Input: dimensioned drawing with shaded views. Units: mm. Origin: part minimum x, y, z. Give positions to 0.01 mm unless a question says otherwise; leave off trailing zeros. Write each loop counter-clockwise with the first axis right and the second up, starting at its lowest first coordinate (ties: lowest second). Pieces come first, ordered by that corner, then holes. Notation, with made-up numbers: (-7, 54.5) -> (10, 54.5) arc R22 ccw to (10, 84.5) -> close; hole circle Ø1 at (62.25, 53.5). An arc over 180 degrees is marked (long way). Answer as a JSON object with one key per item and string values.
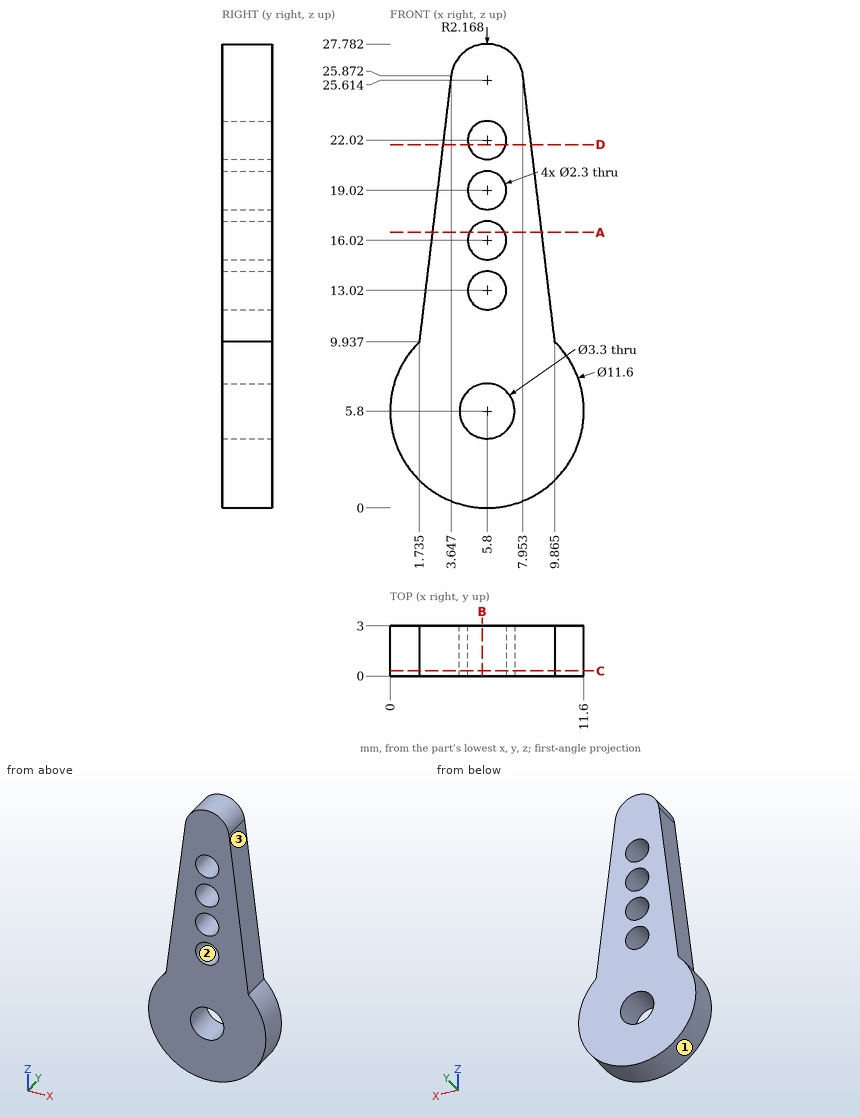
Q1. First-contact query: P1, Ø1.8, axis at x = 5.8, z = 16.02, coming from the -Y side; P2, Ø3.5, axis at x = 5.8, z = 13.02, coming from the -Y side. Flat tips, straight axial feed; report the tip coordinate or a pass-through.
Values:
{"P1": "through", "P2": "y = 0"}
Q2. Material intervals for L1, parallel to Z at x = 5.75, y = 2.35; L2, parallel to Z at x = 7, y = 1.8 (1 decimal); L3, parallel to X at y = 1.8, z = 21.75, sorted ascending. Write a range as from..to.
Values:
{"L1": "0..4.15, 7.45..11.87, 14.17..14.87, 17.17..17.87, 20.17..20.87, 23.17..27.78", "L2": "0.1..4.7, 6.9..27.4", "L3": "3.15..4.68, 6.92..8.45"}
Q3. Mould query, pull axis X, two halves, no side actions, for the marked faces 1, 2 and 3. Classes: pulls with the +X half, pulls with the -X half, needs draft (parallel to the pull), parting line crosses it, or undercut.
Values:
{"face 1": "parting line crosses it", "face 2": "undercut", "face 3": "pulls with the +X half"}
Q4. Cut plane D-D (z = 21.75). Return the cut outline in (x, y).
Values:
{"outline": "(3.15, 0) -> (4.68, 0) -> (4.68, 3) -> (3.15, 3) -> close; (6.92, 0) -> (8.45, 0) -> (8.45, 3) -> (6.92, 3) -> close"}
Q5. Cut plane A-A (z = 16.5). Return the cut outline in (x, y) (1 decimal), and give its area (3 significant figures).
Values:
{"outline": "(2.5, 0) -> (4.8, 0) -> (4.8, 3) -> (2.5, 3) -> close; (6.8, 0) -> (9.1, 0) -> (9.1, 3) -> (6.8, 3) -> close", "area": "13.4 mm²"}
Q6. Cut plane B-B (x = 5.5). Return the cut outline in (y, z).
Values:
{"outline": "(0, 0.01) -> (3, 0.01) -> (3, 4.18) -> (0, 4.18) -> close; (0, 7.42) -> (3, 7.42) -> (3, 11.91) -> (0, 11.91) -> close; (0, 14.13) -> (3, 14.13) -> (3, 14.91) -> (0, 14.91) -> close; (0, 17.13) -> (3, 17.13) -> (3, 17.91) -> (0, 17.91) -> close; (0, 20.13) -> (3, 20.13) -> (3, 20.91) -> (0, 20.91) -> close; (0, 23.13) -> (3, 23.13) -> (3, 27.76) -> (0, 27.76) -> close"}
Q7. Cut plane C-C (y = 0.3). State how many separate pieces and enclosed holes the cut face has.
Values:
{"separate pieces": "1", "enclosed holes": "5"}
